```python
from build123d import *

# Parameters (mm, degrees)
F0_R     = 1.5
F1_DEPTH = 3
F2_W     = 2.2
F2_H     = 2.2
F3_DEPTH = 0.2
F4_W     = 11.4
F4_H     = 2.85
F5_DEPTH = 0.1
F6_W     = 2
F6_H     = 2.85
F7_DEPTH = 0.25


with BuildPart() as f1:
    # F0 (on Top) → F1 (new body)
    with BuildSketch(Plane.XY):
        with BuildLine():
            ThreePointArc((5.053231, 11.711225), (3.778342, 12.753574), (3.24572, 14.311827))
            ThreePointArc((3.24572, 14.311827), (0, 17.395082), (-3.24572, 14.311827))
            ThreePointArc((-3.24572, 14.311827), (-3.778342, 12.753574), (-5.053231, 11.711225))
            ThreePointArc((-5.053231, 11.711225), (-11.046083, 6.377459), (-12.668834, -1.479386))
            ThreePointArc((-12.668834, -1.479386), (-12.93409, -3.104647), (-14.017265, -4.345038))
            ThreePointArc((-14.017265, -4.345038), (-15.14542, -8.548699), (-11.080733, -10.104918))
            Line((-11.080733, -10.104918), (-6.711389, -10.104918))
            Line((-6.711389, -10.104918), (7.566323, -10.104918))
            Line((7.566323, -10.104918), (11.080733, -10.104918))
            ThreePointArc((11.080733, -10.104918), (15.14542, -8.548699), (14.017265, -4.345038))
            ThreePointArc((14.017265, -4.345038), (12.93409, -3.104647), (12.668834, -1.479386))
            ThreePointArc((12.668834, -1.479386), (11.046083, 6.377459), (5.053231, 11.711225))
        make_face()
        with Locations((-12.25, -7.072541)):
            Circle(F0_R, mode=Mode.SUBTRACT)
        with Locations((12.25, -7.072541)):
            Circle(F0_R, mode=Mode.SUBTRACT)
        with Locations((0, 14.145082)):
            Circle(F0_R, mode=Mode.SUBTRACT)
    extrude(amount=F1_DEPTH)

    # F2 (on face) → F3 (join)
    with BuildSketch(Plane.XY.offset(3)):
        with Locations((0, -0.504918)):
            Rectangle(F2_W, F2_H)
    extrude(amount=F3_DEPTH)

    # F4 (on face) → F5 (cut)
    with BuildSketch(Plane.XY.offset(3)):
        with Locations((0, -8.079918)):
            Rectangle(F4_W, F4_H)
    extrude(amount=-F5_DEPTH, mode=Mode.SUBTRACT)

    # F6 (on face) → F7 (join)
    with BuildSketch(Plane.XY.offset(2.9)):
        with Locations((-1.5, -8.079918)):
            Rectangle(F6_W, F6_H)
        with Locations((-4.5, -8.079918)):
            Rectangle(F6_W, F6_H)
        with Locations((1.5, -8.079918)):
            Rectangle(F6_W, F6_H)
        with Locations((4.5, -8.079918)):
            Rectangle(F6_W, F6_H)
    extrude(amount=F7_DEPTH)


solid = f1.part
```
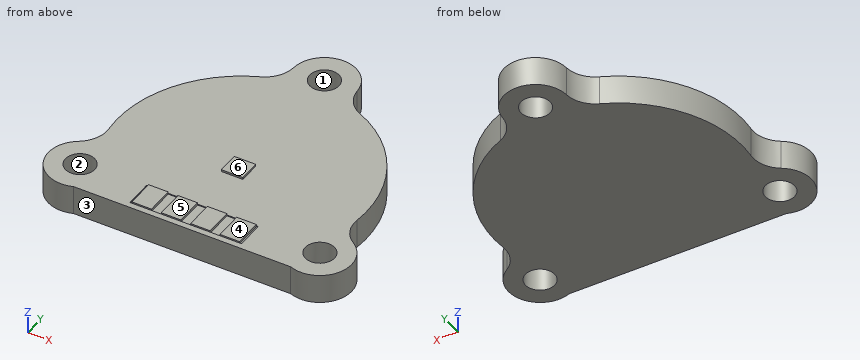
The model under review builds one solid part; all positions refer to its coordinate system, in mm. Face numbers are marked on the shaded views. A direction names the side the tool comes from. Give positions to 0.01 mm unless a question says otherwise; leave off trailing zeros. Write each loop counter-clockwise with the first axis right and the second up, starting at its lowest first coordinate (ties: lowest second). Pieces come first, ordered by that corner, then holes. Notation, with made-up numbers: M -37,46 L 1,46 A8 cw 1,59 Z; hole C -26,43.25 d10. An arc over 180 degrees is marked long. Write each question's results on one line, items separated by ' | '. Start each with the question number.
1. We need section A-A (x = 0). Write out the cut boundary in (y, z), and give its area (3 significant figures).
2. We need section D-D (x = 12). Write out the cut boundary in (y, z).
3. For probe 1 along X at (y, z) = (-6.25, 0.75); probe 2 along Z at (x, y) = (-4.5, 4); probe 3 along Y at (x, z) = (-11, 1.15), list the stretches that pass through material, from the lowest coordinate up. Write a range as [from, to].
4. Mouldability with a two-part tool opening along Y and no side actions: class the marked faces 1, 2, 3 and 4 as released by +Y, released by -Y, zero draft, split by the parting line, or undercut.
5. We need section B-B (z = 1.8). Write out the cut boundary in (x, y).
6. For the marked faces 5 and 6, list the 3-axis set-ups (+Z, -Z, +X, -X, +Y, -Y) from which the entire face can be reached by the end or side of a thin tool; tool diameter is ignored.
7. We need section C-C (y = 13.5). Write out the cut boundary in (x, z), and give its area (3 significant figures).
8. Insertion check: pin 1 Ø2 at (x, y) = (5, -8.5) entering from +Z; pin 2 Ø0.9 at (x, z) = (-2, 2) entering from -Y; pin 3 Ø1.5 at (y, z) = (-2, 1.5) entering from -X. Each pin has a flat end and moves straight along its axis. Give the tip position at first contact, or say it passes through.
Results found:
1) outline: M -10.1,0 L 12.65,0 L 12.65,3 L 0.6,3 L 0.6,3.2 L -1.6,3.2 L -1.6,3 L -6.65,3 L -6.65,2.9 L -9.5,2.9 L -9.5,3 L -10.1,3 Z; M 15.65,0 L 17.4,0 L 17.4,3 L 15.65,3 Z | area: 73.7 mm^2
2) outline: M -10.31,0 L -8.55,0 L -8.55,3 L -10.31,3 Z; M -5.59,0 L 4.32,0 L 4.32,3 L -5.59,3 Z
3) probe 1: x = [-15.39, -13.5], [-11, 11], [13.5, 15.39] | probe 2: z = [0, 3] | probe 3: y = [-10.1, -7.9], [-6.24, 6.46]
4) face 1: undercut | face 2: undercut | face 3: released by -Y | face 4: zero draft
5) outline: M -14.02,-4.35 A3.25 ccw -11.08,-10.1 L 11.08,-10.1 A3.25 ccw 14.02,-4.35 A3 cw 12.67,-1.48 A12.75 ccw 5.05,11.71 A3 cw 3.25,14.31 A3.25 ccw -3.25,14.31 A3 cw -5.05,11.71 A12.75 ccw -12.67,-1.48 A3 cw Z; hole C -12.25,-7.07 d3; hole C 0,14.15 d3; hole C 12.25,-7.07 d3
6) face 5: +Z, +X, -X, -Y | face 6: +Z, +X, -X, +Y, -Y
7) outline: M -3.4,0 L -1.35,0 L -1.35,3 L -3.4,3 Z; M 1.35,0 L 3.4,0 L 3.4,3 L 1.35,3 Z | area: 12.3 mm^2
8) pin 1: stops at z = 3.15 | pin 2: stops at y = -10.1 | pin 3: stops at x = -12.79
